Verification items for the finished model (mm, model axes). A direction names the side the tool comes from. Round coordinates to 2 decimals unless told otherwise and drop trailing zeros. Loops run counter-clockwise (first coordinate to the right, second up) from the corner with the lowest first, then second, coordinate; pieces in that order, holes last.
from build123d import *

# Parameters (mm, degrees)
SKETCH3_R           = 3.5
BOSS_EXTRUDE2_DEPTH = 5.5
SKETCH1_W           = 14.2
SKETCH1_H           = 11.95
BOSS_EXTRUDE3_DEPTH = 3.6
SKETCH4_W           = 7
SKETCH4_H           = 10.45
BOSS_EXTRUDE4_DEPTH = 6


with BuildPart() as part:
    # Sketch3 → Boss-Extrude2 (new body)
    with BuildSketch(Plane(origin=(0, 0, 0), x_dir=(1, 0, 0), z_dir=(0, 1, 0))):
        with Locations(Location((0, 0, 0), (0, 0, 270))):
            Circle(SKETCH3_R)
    extrude(amount=BOSS_EXTRUDE2_DEPTH)

    # Sketch1 → Boss-Extrude3 (add)
    with BuildSketch(Plane(origin=(0, 5.5, 0), x_dir=(1, 0, 0), z_dir=(0, 1, 0))):
        with Locations((3.2, -0.775)):
            Rectangle(SKETCH1_W, SKETCH1_H)
    extrude(amount=BOSS_EXTRUDE3_DEPTH)

    # Sketch4 → Boss-Extrude4 (add)
    with BuildSketch(Plane.XZ.offset(-5.5)):
        with Locations((8.9, 0.425)):
            Rectangle(SKETCH4_W, SKETCH4_H)
    extrude(amount=BOSS_EXTRUDE4_DEPTH)


solid = part.part
1. Section check C-C (x = 8.25). Enter the section's corners in (y, z), then the cut area to 3 significant figures.
2. Section check A-A (y = 5). Enter the section's corners in (x, z), then the cut area to 3 significant figures.
3. Section check D-D (z = 0). Enter the section's corners in (x, y), then the cut area to 3 significant figures.
4. Scan lines: L1, parallel to X at y = 8.25, z = 5; L2, parallel to Z at x = 7, y = 4; L3, parallel to Y at x = -0.5, z = 1.5. Record each from-to range of solid material in increasing order.
5. Section check B-B (z = -3.75). Enter the section's corners in (x, y).
6. Tool access check on faces 4 (the face through (9, 3, -4.8)), 5 (the face through (-3.417, 2.712, -0.759)), 6 (the face through (0, 0, 0)). Record the directions out of +Z, -Z, +X, -X, +Y, -Y that give a thin tool (end or side, any length) a straight path to the whole face; none if there is none.
7. Release check for a two-part mould opening along X. For faces 1 (the face through (-3.9, 7, 1)), 2 (the face through (9, 3, 5.65)), 3 (the face through (3.1, 5.5, 2)) record: released by +X, released by -X, zero draft, split by the parting line, or undercut.
8. Gauge pin test, flat ends, axial feed: P1, Ø3, axis at x = 10.5, y = 2.5, coming from the +Z side; P2, Ø1.7, axis at x = 12, z = -1, coming from the +Y side; P3, Ø3, axis at y = 8, z = -1, coming from the +X side. Record the tip position at first contact, or that the pin passes through.
Taken from the geometry:
1. outline: (-0.5, -4.8) - (5.5, -4.8) - (5.5, -5.2) - (9.1, -5.2) - (9.1, 6.75) - (5.5, 6.75) - (5.5, 5.65) - (-0.5, 5.65) - close
1. area: 106 mm2
2. outline: circle Ø7 at (0, 0); (5.4, -4.8) - (12.4, -4.8) - (12.4, 5.65) - (5.4, 5.65) - close
2. area: 112 mm2
3. outline: (-3.9, 5.5) - (-3.5, 5.5) - (-3.5, 0) - (3.5, 0) - (3.5, 5.5) - (5.4, 5.5) - (5.4, -0.5) - (12.4, -0.5) - (12.4, 5.5) - (10.3, 5.5) - (10.3, 9.1) - (-3.9, 9.1) - close
3. area: 132 mm2
4. L1: x = -3.9 to 10.3
4. L2: z = -4.8 to 5.65
4. L3: y = 0 to 9.1
5. outline: (-3.9, 5.5) - (5.4, 5.5) - (5.4, -0.5) - (12.4, -0.5) - (12.4, 5.5) - (10.3, 5.5) - (10.3, 9.1) - (-3.9, 9.1) - close
6. face 4: -Z, +X, -X, -Y
6. face 5: -Y
6. face 6: +Z, -Z, -X, -Y
7. face 1: released by -X
7. face 2: zero draft
7. face 3: undercut
8. P1: stops at z = 5.65
8. P2: stops at y = 5.5
8. P3: stops at x = 10.3
